The listing builds one solid part. Answer for the finished solid, in the listing's coordinates (mm). A direction names the side the tool comes from. Round coordinates to 2 decimals unless told otherwise and drop trailing zeros. Loops run counter-clockwise (first coordinate to the right, second up) from the corner with the lowest first, then second, coordinate; pieces in that order, holes last. Notation, with made-up numbers: (65.25, -15) - (112.25, -15) arc R17 cw to (112.25, 9) - close; hole circle Ø1 at (-12.75, 48). An arc over 180 degrees is marked (long way). Write item = value, one per line. Start each with the question number.
1) Section A-A, the plane x = -10.5 is taken. Determine the outline of the cut face in (y, z), and give its area (3 significant figures).
2) Given pin 1 Ø1.5 at (x, z) = (-29, 2) entering from +Y; pin 2 Ø1 at (x, y) = (-54.5, -3) entering from -Z, each flat-ended and moving along its own axis, determine where each tip first touches the part or whether it passes through.
3) A tool of negligible diameter and unlimited length cuts with its end or side. For faces 1 (the flat face through (0, 1, 3)), 2 (the flat face through (2.737, 0, 0)), from which of +Z, -Z, +X, -X, +Y, -Y can it reach the whole face along a straight path? Write none if from no direction.
4) Straight lines are drawn through the part: line 1 along X through (y, z) = (2.5, 2); line 2 along X through (y, z) = (-3, -2.5); line 3 along Y through (x, z) = (-56, 0.25). For each, find the intervals that lie inside material, in ascending order.
from build123d import *

# Parameters (mm, degrees)
CHAMFER1_SIZE = 0.5


with BuildPart() as part:
    # Sketch1 → Revolve1 (revolve)
    with BuildSketch(Plane.XY):
        Polygon((0.7366, 4), (2.7366, 4), (2.7366, 0), (-132.2634, 0), (-132.2634, 4), (0, 4), (0, 3), (0.7366, 3), align=None)
    revolve(axis=Axis((2.7366, 0, 0), (1, 0, 0)))

    # Chamfer1
    chamfer1_edges = [part.edges().sort_by_distance(p)[0] for p in [
        (2.7366, -4, 0),
        (-132.2634, -4, 0),
    ]]
    chamfer(chamfer1_edges, length=CHAMFER1_SIZE)


solid = part.part
Geometry check:
q1.outline = circle Ø8 at (0, 0)
q1.area = 50.3 mm2
q2.pin_1 = 3.8
q2.pin_2 = -3.12
q3.face_1 = none
q3.face_2 = +Z, -Z, +X, +Y, -Y
q4.line_1 = -132.26 to 0, 0.74 to 2.74
q4.line_2 = -131.86 to 0, 0.74 to 2.33
q4.line_3 = -3.99 to 3.99
